from build123d import *

# Parameters (mm, degrees)
SKETCH4_R           = 20
BOSS_EXTRUDE2_DEPTH = 3
SKETCH5_R           = 19
BOSS_EXTRUDE3_DEPTH = 9
SKETCH6_R           = 13
BOSS_EXTRUDE4_DEPTH = 17
SKETCH7_R           = 18
CUT_EXTRUDE3_DEPTH  = 10
SKETCH8_R           = 10
CUT_EXTRUDE4_DEPTH  = 19
BOSS_EXTRUDE5_DEPTH = 26
SKETCH10_R          = 13
CUT_EXTRUDE5_DEPTH  = 10
SKETCH11_R          = 9
CUT_EXTRUDE6_DEPTH  = 26
CUT_EXTRUDE7_START  = -10
SKETCH12_R          = 13
CUT_EXTRUDE7_DEPTH  = 10
CUT_EXTRUDE8_START  = -20
SKETCH13_R          = 9
CUT_EXTRUDE8_DEPTH  = 20
CUT_EXTRUDE15_DEPTH = 10.15


with BuildPart() as part:
    # Sketch4 → Boss-Extrude2 (new body)
    with BuildSketch(Plane(origin=(0, 0, 0), x_dir=(1, 0, 0), z_dir=(0, 1, 0))):
        with Locations(Location((0, 0, 0), (0, 0, 270))):
            Circle(SKETCH4_R)
    extrude(amount=-BOSS_EXTRUDE2_DEPTH)

    # Sketch5 → Boss-Extrude3 (add)
    with BuildSketch(Plane.XZ.offset(3)):
        with Locations(Location((0, 0, 0), (0, 0, 270))):
            Circle(SKETCH5_R)
    extrude(amount=BOSS_EXTRUDE3_DEPTH)

    # Sketch6 → Boss-Extrude4 (add)
    with BuildSketch(Plane.XZ.offset(12)):
        with Locations(Location((0, 0, 0), (0, 0, 270))):
            Circle(SKETCH6_R)
    extrude(amount=BOSS_EXTRUDE4_DEPTH)

    # Sketch7 → Cut-Extrude3 (cut)
    with BuildSketch(Plane(origin=(0, 0, 0), x_dir=(1, 0, 0), z_dir=(0, 1, 0))):
        with Locations(Location((0, 0, 0), (0, 0, 270))):
            Circle(SKETCH7_R)
    extrude(amount=-CUT_EXTRUDE3_DEPTH, mode=Mode.SUBTRACT)

    # Sketch8 → Cut-Extrude4 (cut)
    with BuildSketch(Plane.XZ.offset(29)):
        with Locations(Location((0, 0, 0), (0, 0, 270))):
            Circle(SKETCH8_R)
    extrude(amount=-CUT_EXTRUDE4_DEPTH, mode=Mode.SUBTRACT)

    # Sketch9 → Boss-Extrude5 (add, symmetric)
    with BuildSketch(Plane.XY):
        Polygon((0, -17), (-18, -27.392304845), (-18, -48.176914536), (0, -58.569219382), (18, -48.176914536), (18, -27.392304845), align=None)
    extrude(amount=BOSS_EXTRUDE5_DEPTH, both=True)

    # Sketch10 → Cut-Extrude5 (cut)
    with BuildSketch(Plane.XY.offset(26)):
        with Locations((0, -37.784609691)):
            Circle(SKETCH10_R)
    extrude(amount=-CUT_EXTRUDE5_DEPTH, mode=Mode.SUBTRACT)

    # Sketch11 → Cut-Extrude6 (cut)
    with BuildSketch(Plane.XY.offset(16)):
        with Locations((0, -37.784609691)):
            Circle(SKETCH11_R)
    extrude(amount=-CUT_EXTRUDE6_DEPTH, mode=Mode.SUBTRACT)

    # Sketch12 → Cut-Extrude7 (cut)
    with BuildSketch(Plane(origin=(0, 0, -26), x_dir=(-1, 0, 0), z_dir=(0, 0, -1)).offset(CUT_EXTRUDE7_START)):
        with Locations(Location((0, -37.784609691, 0), (0, 0, 180))):
            Circle(SKETCH12_R)
    extrude(amount=CUT_EXTRUDE7_DEPTH, mode=Mode.SUBTRACT)

    # Sketch13 → Cut-Extrude8 (cut)
    with BuildSketch(Plane(origin=(0, 0, -16), x_dir=(-1, 0, 0), z_dir=(0, 0, -1)).offset(CUT_EXTRUDE8_START)):
        with Locations(Location((0, -37.784609691, 0), (0, 0, 180))):
            Circle(SKETCH13_R)
    extrude(amount=CUT_EXTRUDE8_DEPTH, mode=Mode.SUBTRACT)

    # Sketch30 → Cut-Extrude15 (cut, symmetric)
    with BuildSketch(Plane(origin=(0, 0, 0), x_dir=(0, 0, -1), z_dir=(1, 0, 0))):
        with BuildLine():
            Line((-15.826629517, -58.510939608), (15.298060877, -58.510939608))
            ThreePointArc((15.298060877, -58.510939608), (13.502204004, -55.924078568), (10.390732376, -55.438592985))
            ThreePointArc((10.390732376, -55.438592985), (0.01479369, -56.801466399), (-10.38951563, -55.675466788))
            ThreePointArc((-10.38951563, -55.675466788), (-13.769795356, -55.824327649), (-15.826629517, -58.510939608))
        make_face()
    extrude(amount=CUT_EXTRUDE15_DEPTH, both=True, mode=Mode.SUBTRACT)

    # Sketch36 → Cut-Revolve2 (revolve, cut)
    with BuildSketch(Plane(origin=(0, 0, 0), x_dir=(0, 0, -1), z_dir=(1, 0, 0))):
        with BuildLine():
            Line((-7, -52.801466399), (0, -52.801466399))
            Line((0, -52.801466399), (0, -17))
            Line((0, -17), (-10, -17))
            Line((-10, -17), (-10, -27))
            Line((-10, -27), (-9, -28.785233738))
            Line((-9, -28.785233738), (-7, -49))
            ThreePointArc((-7, -49), (-7.678962882, -50.900733199), (-7, -52.801466399))
        make_face()
    revolve(axis=Axis((0, -17, 0), (0, -1, 0)), mode=Mode.SUBTRACT)


solid = part.part
The model under review builds one solid part; all positions refer to its coordinate system, in mm. A direction names the side the tool comes from. Round coordinates to 2 decimals unless told otherwise and drop trailing zeros. Order: outer loops, then holes, each group sorted by start corner. A loop starts at its lowest first (then second) coordinate and runs counter-clockwise, first axis right, second up. Notation, with made-up numbers: (-8, 17.25) -> (35, 17.25) arc R20 cw to (35, 50.25) -> close; hole circle Ø4 at (13, -40). An arc over 180 degrees is marked (long way). Return JSON: item names as keys, results as strings.
1. Take a section at D-D (y = -14.5). Write out the cut boundary in (x, z), then the cut area to 3 significant figures.
Answer block:
{"outline": "circle Ø26 at (0, 0); hole circle Ø20 at (0, 0)", "area": "217 mm²"}
2. Take a section at A-A (z = 15). Write out the cut boundary in (x, y), then the cut area to 3 significant figures.
Answer block:
{"outline": "(-18, -48.18) -> (-3.03, -56.82) -> (3.03, -56.82) -> (18, -48.18) -> (18, -27.39) -> (0, -17) -> (-18, -27.39) -> close; (-13.23, -3) -> (-11.66, -3) -> (-11.66, -12) -> (11.66, -12) -> (11.66, -3) -> (13.23, -3) -> (13.23, 0) -> (9.95, 0) -> (9.95, -10) -> (-9.95, -10) -> (-9.95, 0) -> (-13.23, 0) -> close; (-0.1, -58.51) -> (0, -58.57) -> (0.1, -58.51) -> close; hole circle Ø18 at (0, -37.78)", "area": "953 mm²"}
3. The part is to be moulded in two halves that separate along Z. For faces 1 (the face through (-11.56, -7.44, 15.08)), 2 (the face through (-14.874, -25.588, 0.364)), 3 (the face through (-8.77, -31.09, 0.19)), say which applies: +Z half, -Z half, draft (parallel to the pull), parting line (faces both ways), or undercut.
Answer block:
{"face 1": "parting line", "face 2": "draft", "face 3": "undercut"}
4. Take a section at C-C (y = -45). Write out the cut boundary in (x, z).
Answer block:
{"outline": "(-18, -26) -> (-10.81, -26) -> (-10.81, -16) -> (-5.38, -16) -> (-5.38, -5.08) arc R7.4 cw to (-5.38, 5.08) -> (-5.38, 16) -> (-10.81, 16) -> (-10.81, 26) -> (-18, 26) -> close; (5.38, -16) -> (10.81, -16) -> (10.81, -26) -> (18, -26) -> (18, 26) -> (10.81, 26) -> (10.81, 16) -> (5.38, 16) -> (5.38, 5.08) arc R7.4 cw to (5.38, -5.08) -> close"}
5. Take a section at B-B (x = -15). Write out the cut boundary in (y, z), then the cut area to 3 significant figures.
Answer block:
{"outline": "(-49.91, -26) -> (-25.66, -26) -> (-25.66, 26) -> (-49.91, 26) -> close; (-12, -11.66) -> (-3, -11.66) -> (-3, -13.23) -> (0, -13.23) -> (0, -9.95) -> (-10, -9.95) -> (-10, 9.95) -> (0, 9.95) -> (0, 13.23) -> (-3, 13.23) -> (-3, 11.66) -> (-12, 11.66) -> close", "area": "1,350 mm²"}
6. For faces 4 (the face through (-2.818, -25.094, -20.93)), 5 (the face through (-9.582, -28.999, 21.07)), 6 (the face through (18, -38, 0)), 7 (the face through (-8, -10, 8)), list the 3-axis set-ups (+Z, -Z, +X, -X, +Y, -Y) from which the entire face can be reached by the end or side of a thin tool; tool diameter is ignored.
Answer block:
{"face 4": "-Z", "face 5": "+Z", "face 6": "+Z, -Z, +X, -Y", "face 7": "+Y"}
7. For L1, parallel to Y at x = 0, z = 19.5; L2, parallel to Y at x = 0, z = 23; L3, parallel to Y at x = -7, z = 11, list the stretches that pass through material, from the lowest coordinate up. Write a range as [from, to].
Answer block:
{"L1": "y = [-58.57, -50.78], [-24.78, -17], [-3, 0]", "L2": "y = [-58.57, -50.78], [-24.78, -17]", "L3": "y = [-54.53, -43.44], [-32.13, -21.04], [-12, -10]"}
8. Insertion check: P1, Ø11, axis at x = -1, z = 1, coming from the +Y side; P2, Ø10.5, axis at y = -39.5, z = 12.5, coming from the -X side; P3, Ø11.5, axis at x = -8, z = -6, coming from the -Y side; P4, Ø12, axis at x = 11, z = -18.5, coming from the +Y side. Each pin has a flat end and moves straight along its axis. Give the tip position at first contact, or say it passes through.
Answer block:
{"P1": "stops at y = -52.8", "P2": "stops at x = -18", "P3": "stops at y = -56.69", "P4": "stops at y = 0"}
